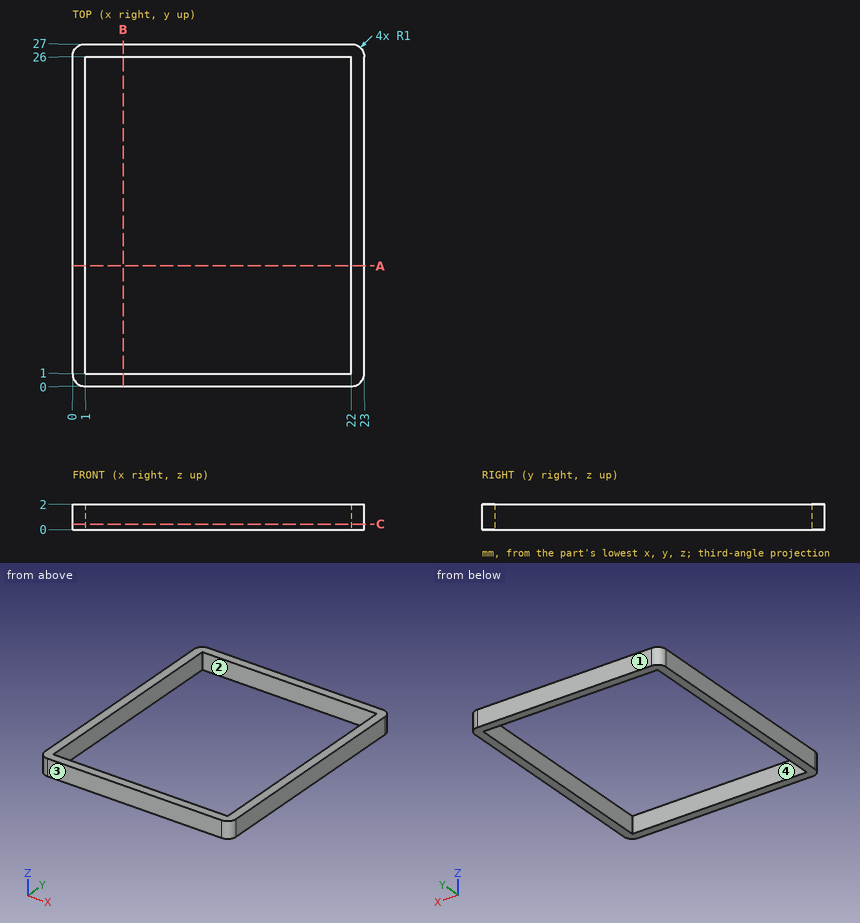
Could you check a few things on this drawing? It's one solid part, dimensions in mm from its lowest x, y, z. A direction names the side the tool comes from. Coordinates: 2 decimals unless noted, no trailing zeros. Order: outer loops, then holes, each group sorted by start corner. A loop starts at its lowest first (then second) coordinate and runs counter-clockwise, first axis right, second up. Notation, with made-up numbers: M 20.5,6.25 L 24.5,6.25 A27 ccw 24.5,25.25 Z; hole C 79.5,-21.75 d11. An arc over 180 degrees is marked long. Use a Markdown table: item, result. Add a question column.
Q1. We'd pull the mould along X, two halves only. Please class the marked faces 3 and 4: pulls with the +X half, pulls with the -X half, needs draft (parallel to the pull), parting line crosses it, or undercut.
Q2. Which directions (+Z, -Z, +X, -X, +Y, -Y) give clear straight access to the entire face, cutting with the end or side of a thin tool? Please do the marked faces 1 and 2.
Q3. I'm going to push a flat-ended pin straight in: pin 1 (4 mm diameter, centred on x = 3.5, y = 16.5, fed in from +Z). Where does the tip first touch, or does it pass through?
Q4. I want a section at C-C on z = 0.45. List the corners of the cut face in (x, y) for me.
Q5. If I drill on L1, parallel to X at y = 21.5, z = 0.2; L2, parallel to Y at x = 13.5, z = 1.85, over which ranges is the centre line in solid material (lowest first)?
Q6. I want a section at A-A on y = 9.5. List the corners of the cut face in (x, z) for me.
Q7. I want a section at B-B on x = 4. List the corners of the cut face in (y, z) for me.
Checked values:
| question | item | result |
|---|---|---|
| 1 | face 3 | needs draft |
| 1 | face 4 | undercut |
| 2 | face 1 | +Z, -Z, +X, -X, +Y |
| 2 | face 2 | +Z, -Z |
| 3 | pin 1 | through |
| 4 | outline | M 0,1 A1 ccw 1,0 L 22,0 A1 ccw 23,1 L 23,26 A1 ccw 22,27 L 1,27 A1 ccw 0,26 Z; hole M 1,1 L 22,1 L 22,26 L 1,26 Z |
| 5 | L1 | 0 to 1, 22 to 23 |
| 5 | L2 | 0 to 1, 26 to 27 |
| 6 | outline | M 0,0 L 1,0 L 1,2 L 0,2 Z; M 22,0 L 23,0 L 23,2 L 22,2 Z |
| 7 | outline | M 0,0 L 1,0 L 1,2 L 0,2 Z; M 26,0 L 27,0 L 27,2 L 26,2 Z |
